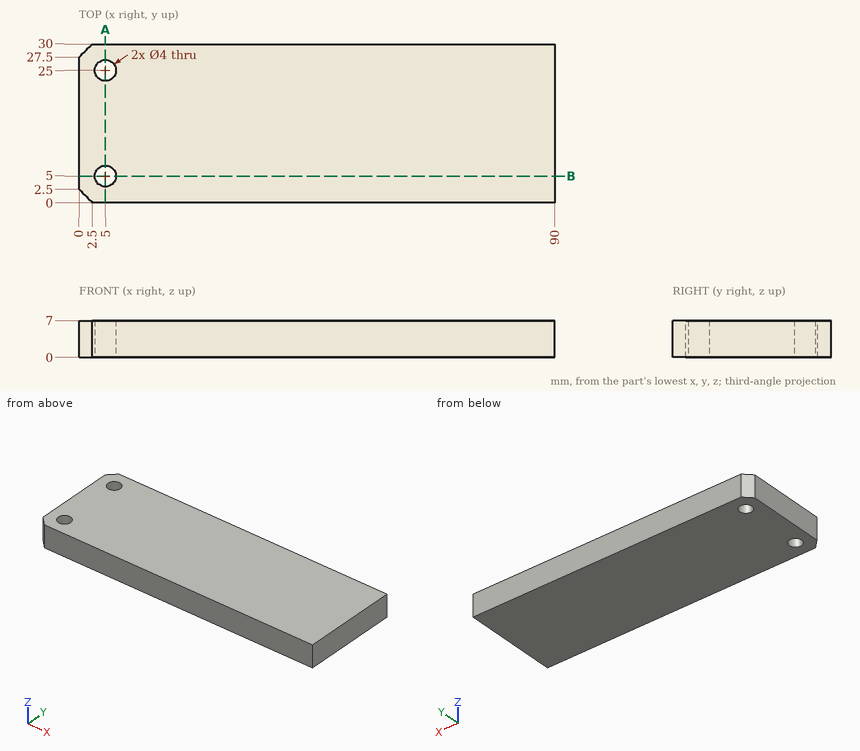
Part print with two shaded views. Sizes in mm from the minimum x, y, z corner. Give positions to 0.01 mm unless a question says otherwise; leave off trailing zeros. Order: outer loops, then holes, each group sorted by start corner. A loop starts at its lowest first (then second) coordinate and runs counter-clockwise, first axis right, second up.
(1) Saw through at B-B, the plane y = 5. Give the cut face in (x, z).
(2) Saw through at A-A, the plane x = 5. Give the cut face in (y, z).
(3) Drill centre lines: L1, parallel to Y at x = 5, z = 2; L2, parallel to X at y = 5, z = 3.5; L3, parallel to Y at x = 6, z = 2.5. Where is each one in solid material? Low to high.
Results found:
1. outline: (0, 0) - (3, 0) - (3, 7) - (0, 7) - close; (7, 0) - (90, 0) - (90, 7) - (7, 7) - close
2. outline: (0, 0) - (3, 0) - (3, 7) - (0, 7) - close; (7, 0) - (23, 0) - (23, 7) - (7, 7) - close; (27, 0) - (30, 0) - (30, 7) - (27, 7) - close
3. L1: y = 0 to 3, 7 to 23, 27 to 30
3. L2: x = 0 to 3, 7 to 90
3. L3: y = 0 to 3.27, 6.73 to 23.27, 26.73 to 30
